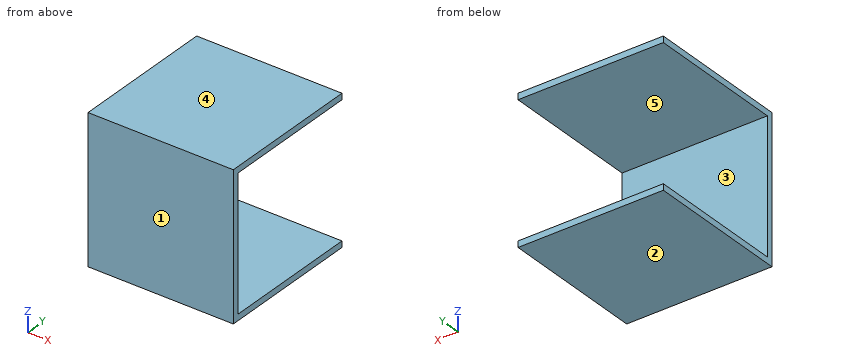
Autodesk Inventor part; units mm, degrees
ref_plane "YZ Plane" through (0, 0, 0) normal (1, 0, 0) x (0, 1, 0)
ref_plane "XZ Plane" through (0, 0, 0) normal (0, 1, 0) x (-1, 0, 0)
ref_plane "XY Plane" through (0, 0, 0) normal (0, 0, 1) x (1, 0, 0)
sketch "Sketch1" plane through (0, 0, 0) normal (0, 1, 0) x (-1, 0, 0)
  line L0 (93.0994, 142.6523) -> (-206.6206, 142.6523)
  line L1 (-206.6206, 142.6523) -> (-206.6206, -157.0677)
  line L2 (-206.6206, -157.0677) -> (93.0994, -157.0677)
  line L3 (93.0994, -157.0677) -> (93.0994, 142.6523)
  point P0 (0, 0)
  dimension "d0" = 299.72
  dimension "d1" = 299.72
extrude "Extrusion1" add sketch "Sketch1" along normal blind 12.7
sketch "Sketch2" plane through (0, 12.7, 0) normal (0, 1, 0) x (1, 0, 0)
  line L0 (-93.0994, -142.6523) -> (206.6206, -142.6523)
  line L1 (206.6206, -142.6523) -> (206.6206, 157.0677)
  line L2 (-93.0994, -142.6523) -> (206.6206, -142.6523)
  line L3 (206.6206, -142.6523) -> (206.6206, -129.9523)
  line L4 (206.6206, -129.9523) -> (-93.0994, -129.9523)
  line L5 (-93.0994, -129.9523) -> (-93.0994, -142.6523)
  point P0 (0, 0)
  dimension "d4" = 12.7
extrude "Extrusion2" add sketch "Sketch2" along normal blind 287.02
sketch "Sketch3" plane through (0, 12.7, 0) normal (0, 1, 0) x (1, 0, 0)
  line L0 (-93.0994, 157.0677) -> (-93.0994, -129.9523)
  line L1 (206.6206, -129.9523) -> (206.6206, 157.0677)
  line L2 (-93.0994, 157.0677) -> (206.6206, 157.0677)
  line L3 (206.6206, 157.0677) -> (206.6206, 144.3677)
  line L4 (206.6206, 144.3677) -> (-93.0994, 144.3677)
  line L5 (-93.0994, 144.3677) -> (-93.0994, 157.0677)
  point P0 (0, 0)
  dimension "d7" = 12.7
extrude "Extrusion3" add sketch "Sketch3" along normal blind 287.02
properties part number "chassisFloor"
Here's how the part is built. I have some questions about the finished solid (model axes, mm). Face numbers are marked on the shaded views. A direction names the side the tool comes from. Coordinates: 2 decimals unless noted, no trailing zeros. Loops run counter-clockwise (first coordinate to the right, second up) from the corner with the lowest first, then second, coordinate; pieces in that order, holes last. Notation, with made-up numbers: (-12.75, 68.5) - (15.25, 68.5) arc R14 cw to (15.25, 89.5) - close; hole circle Ø2 at (15, -37). An arc over 180 degrees is marked (long way). Answer as CSV lines item,"result".
Q1. If we section it at C-C, the plane z = -101.5: Write out the boundary of the cut face in (x, y), and give its area (3 significant figures).
Response:
outline,"(-93.1, 0) - (206.62, 0) - (206.62, 12.7) - (-93.1, 12.7) - close"
area,"3,810 mm2"
Q2. For the marked faces 4 and 5, which set-ups out of +Z, -Z, +X, -X, +Y, -Y let a thin tool reach every point of the face, with its end or its side?
Response:
face 4,"+Z, +X, -X, +Y, -Y"
face 5,"+X, -X, +Y"
Q3. For pin 1 (1.5 mm diameter, centred on x = 58.5, z = 98, fed in from +Y), with a flat end and sliding along its axis, tell me the tip position at first contact or that it passes through.
Response:
pin 1,"y = 12.7"
Q4. If I drill on L1, parallel to Z at x = 78, y = 118; L2, parallel to Y at x = 101.5, z = 37, over which ranges is the centre line in solid material (lowest first)? Write a range as [from, to].
Response:
L1,"[-157.07, -144.37], [129.95, 142.65]"
L2,"[0, 12.7]"
Q5. We'd pull the mould along Z, two halves only. Please class the marked faces 1, 2 and 3: pulls with the +Z half, pulls with the -Z half, needs draft (parallel to the pull), parting line crosses it, or undercut.
Response:
face 1,"needs draft"
face 2,"pulls with the -Z half"
face 3,"undercut"
Q6. If we section it at B-B, the plane x = 126: Write out the boundary of the cut face in (y, z).
Response:
outline,"(0, -157.07) - (299.72, -157.07) - (299.72, -144.37) - (12.7, -144.37) - (12.7, 129.95) - (299.72, 129.95) - (299.72, 142.65) - (0, 142.65) - close"
Q7. If we section it at A-A, the plane y = 264.5: Write out the boundary of the cut face in (x, z).
Response:
outline,"(-93.1, -157.07) - (206.62, -157.07) - (206.62, -144.37) - (-93.1, -144.37) - close; (-93.1, 129.95) - (206.62, 129.95) - (206.62, 142.65) - (-93.1, 142.65) - close"
